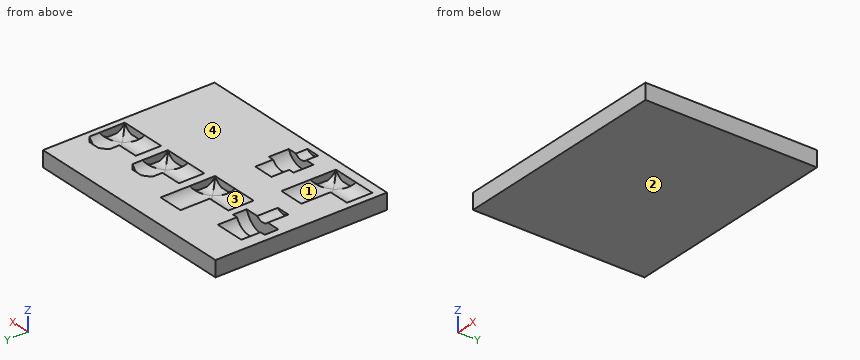
from build123d import *

# Parameters (mm, degrees)
F0_W      = 160
F0_H      = 125
F1_DEPTH  = 16.5
F4_W      = 35
F4_H      = 10.5
F6_W      = 37
F6_H      = 10.5
F8_W      = 10.5
F8_H      = 20
F8_H_2    = 21
F10_W     = 35
F10_H     = 10.5
F12_W     = 10.5
F12_H     = 21
F14_W     = 10.5
F14_H     = 21
F16_W     = 10.5
F16_H     = 20
F16_H_2   = 21
F20_W     = 160
F20_H     = 5
F21_DEPTH = 160
F22_W     = 1.2669073437
F22_H     = 18.4661853126
F22_W_2   = 18.4661853126
F22_H_2   = 1.2669073437
F23_DEPTH = 5


with BuildPart() as f1:
    # F0 (on Top) → F1 (new body)
    with BuildSketch(Plane.XY):
        with Locations((80, 62.5)):
            Rectangle(F0_W, F0_H)
    extrude(amount=-F1_DEPTH)

    # F2 (on face) → F3 (revolve, cut)
    with BuildSketch(Plane.XY):
        Polygon((20, 75), (20, 60), (27, 60), (27, 75), (35.5, 75), (35.5, 85), (32, 85), (32, 99), (24.5, 99), (24.5, 113), (20, 113), (20, 99), (20, 85), align=None)
    revolve(axis=Axis((20, 92, 0), (0, 1, 0)), mode=Mode.SUBTRACT)

    # F4 (on face) → F5 (revolve, cut)
    with BuildSketch(Plane.XY):
        with Locations((22.5, 10.75)):
            Rectangle(F4_W, F4_H)
    revolve(axis=Axis((22.5, 16, 0), (1, 0, 0)), mode=Mode.SUBTRACT)

    # F6 (on face) → F7 (revolve, cut)
    with BuildSketch(Plane.XY):
        with Locations((58.5, 69.75)):
            Rectangle(F6_W, F6_H)
    revolve(axis=Axis((58.5, 75, 0), (1, 0, 0)), mode=Mode.SUBTRACT)

    # F8 (on face) → F9 (revolve, cut)
    with BuildSketch(Plane.XY):
        with Locations((71.75, 95.5)):
            Rectangle(F8_W, F8_H)
        with Locations((71.75, 75)):
            Rectangle(F8_W, F8_H_2)
    revolve(axis=Axis((66.5, 85, 0), (0, 1, 0)), mode=Mode.SUBTRACT)

    # F10 (on face) → F11 (revolve, cut)
    with BuildSketch(Plane.XY):
        with Locations((99.5, 72.75)):
            Rectangle(F10_W, F10_H)
        with Locations((139.5, 72.75)):
            Rectangle(F10_W, F10_H)
    revolve(axis=Axis((99.5, 78, 0), (1, 0, 0)), mode=Mode.SUBTRACT)

    # F12 (on face) → F13 (revolve, cut)
    with BuildSketch(Plane.XY):
        Polygon((106.5, 88.5), (117, 88.5), (117, 94.5), (113, 98.5), (106.5, 98.5), align=None)
        with Locations((111.75, 78)):
            Rectangle(F12_W, F12_H)
    revolve(axis=Axis((106.5, 83, 0), (0, 1, 0)), mode=Mode.SUBTRACT)

    # F14 (on face) → F15 (revolve, cut)
    with BuildSketch(Plane.XY):
        Polygon((146.5, 88.5), (157, 88.5), (157, 94.5), (153, 98.5), (146.5, 98.5), align=None)
        with Locations((151.75, 78)):
            Rectangle(F14_W, F14_H)
    revolve(axis=Axis((146.5, 83, 0), (0, 1, 0)), mode=Mode.SUBTRACT)

    # F16 (on face) → F17 (revolve, cut)
    with BuildSketch(Plane.XY):
        with Locations((34.75, 36.5)):
            Rectangle(F16_W, F16_H)
        with Locations((34.75, 16)):
            Rectangle(F16_W, F16_H_2)
    revolve(axis=Axis((29.5, 26, 0), (0, 1, 0)), mode=Mode.SUBTRACT)

    # F18 (on face) → F19 (revolve, cut)
    with BuildSketch(Plane.XY):
        Polygon((62.5, 13.5), (62.5, 5), (69.5, 5), (69.5, 13.5), (75, 13.5), (75, 28), (71.5, 28), (71.5, 41), (62.5, 41), (62.5, 28), align=None)
    revolve(axis=Axis((62.5, 20.75, 0), (0, 1, 0)), mode=Mode.SUBTRACT)

    # F20 (on face) → F21 (cut)
    with BuildSketch(Plane.XZ):
        with Locations((80, -2.5)):
            Rectangle(F20_W, F20_H)
    extrude(amount=-F21_DEPTH, mode=Mode.SUBTRACT)

    # F22 (on face) → F23 (join)
    with BuildSketch(Plane.XY.offset(-5)):
        with Locations((39.3665463282, 16)):
            Rectangle(F22_W, F22_H)
        with Locations((29.5, 6.1334536718)):
            Rectangle(F22_W_2, F22_H_2)
        with Locations((76.3665463282, 75)):
            Rectangle(F22_W, F22_H)
        with Locations((66.5, 65.1334536718)):
            Rectangle(F22_W_2, F22_H_2)
        with Locations((116.3665463282, 78)):
            Rectangle(F22_W, F22_H)
        with Locations((106.5, 68.1334536718)):
            Rectangle(F22_W_2, F22_H_2)
        with Locations((156.3665463282, 78)):
            Rectangle(F22_W, F22_H)
        with Locations((146.5, 68.1334536718)):
            Rectangle(F22_W_2, F22_H_2)
    extrude(amount=-F23_DEPTH)


solid = f1.part
Verification items for the finished model (mm, model axes). Face numbers are marked on the shaded views. A direction names the side the tool comes from. Give positions to 0.01 mm unless a question says otherwise; leave off trailing zeros. Loops run counter-clockwise (first coordinate to the right, second up) from the corner with the lowest first, then second, coordinate; pieces in that order, holes last. Notation, with made-up numbers: (87, 8) - (120, 8) arc R33 ccw to (120, 38) - close; hole circle Ø1 at (-22, 37.5). An arc over 180 degrees is marked (long way). Write item = value, one per line. Start each with the question number.
Q1. Tool access check on the marked faces 3 and 4. Record the directions out of +Z, -Z, +X, -X, +Y, -Y that give a thin tool (end or side, any length) a straight path to the whole face; none if there is none.
Q2. Mould release check, pull along Y, two halves, no side actions. Record for the marked faces 1 and 2: released by +Y, released by -Y, zero draft, split by the parting line, or undercut.
Q3. Cross-section at B-B, the plane y = 23. Enter the section's corners in (x, z), and give its area (3 significant figures).
Q4. Cross-section at C-C, the plane y = 9. Enter the section's corners in (x, z).
Q5. Cross-section at A-A, the plane y = 36. Enter the section's corners in (x, z), and give its area (3 significant figures).
Q6. Thickness scan on line 1 (X direction, y = 74, z = -7.5); line 2 (Y direction, x = 67.5, z = -6); line 3 (Y direction, x = 26, z = -12). Record the ranges inside material, lowest first.
Answer key:
q1.face_3 = +Z
q1.face_4 = +Z, +X, -X, +Y, -Y
q2.face_1 = undercut
q2.face_2 = zero draft
q3.outline = (0, -16.5) - (160, -16.5) - (160, -5) - (73.96, -5) arc R12.5 cw to (51.04, -5) - (38.73, -5) - (38.73, -7.83) - (36.5, -7.83) arc R10.5 cw to (22.5, -7.83) - (5, -7.83) - (5, -5) - (0, -5) - close
q3.area = 1,600 mm^2
q4.outline = (0, -16.5) - (160, -16.5) - (160, -5) - (67.4, -5) arc R7 cw to (57.6, -5) - (38.73, -5) - (38.73, -7.83) - (36.5, -7.83) arc R10.5 cw to (22.5, -7.83) - (5, -7.83) - (5, -5) - (0, -5) - close
q5.outline = (0, -16.5) - (160, -16.5) - (160, -5) - (69.98, -5) arc R9 cw to (55.02, -5) - (38.73, -5) arc R10.5 cw to (20.27, -5) - (0, -5) - close
q5.area = 1,730 mm^2
q6.line_1 = 0 to 40, 75.73 to 82, 115.73 to 122, 155.73 to 160
q6.line_2 = 0 to 13.5, 41 to 65.77, 105.5 to 125
q6.line_3 = 0 to 75, 85 to 125
